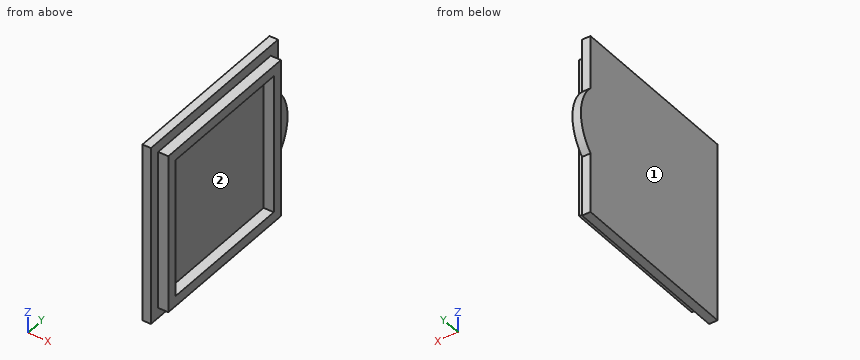
Autodesk Inventor part; units mm, degrees
ref_plane "YZ Plane" through (0, 0, 0) normal (1, 0, 0) x (0, 1, 0)
ref_plane "XZ Plane" through (0, 0, 0) normal (0, 1, 0) x (-1, 0, 0)
ref_plane "XY Plane" through (0, 0, 0) normal (0, 0, 1) x (1, 0, 0)
sketch "Skizze4" plane through (0, 0, 0) normal (1, 0, 0) x (0, 1, 0)
  line L0 (26.5, 26.5) -> (-26.5, 26.5)
  line L1 (-26.5, 26.5) -> (-26.5, -26.5)
  line L2 (-26.5, -26.5) -> (26.5, -26.5)
  line L3 (26.5, -26.5) -> (26.5, 26.5)
  line L4 (0, -37.1) -> (0, 37.1) construction
  line L5 (-37.1, 0) -> (37.1, 0) construction
  dimension "d18" = 53
  dimension "d19" = 53
extrude "Extrusion2" add sketch "Skizze4" along normal blind 2.5
sketch "Skizze5" plane through (2.5, 0, 0) normal (1, 0, 0) x (0, 0, -1)
  line L0 (-26.5, -26.5) -> (26.5, -26.5) construction
  line L1 (26.5, -26.5) -> (26.5, 26.5) construction
  line L2 (26.5, 26.5) -> (-26.5, 26.5) construction
  line L3 (-26.5, 26.5) -> (-26.5, -26.5) construction
  line L4 (-23.5, 23.5) -> (23.5, 23.5)
  line L5 (23.5, 23.5) -> (23.5, -23.5)
  line L6 (23.5, -23.5) -> (-23.5, -23.5)
  line L7 (-23.5, -23.5) -> (-23.5, 23.5)
  line L8 (20.5, 20.5) -> (-20.5, 20.5)
  line L9 (-20.5, 20.5) -> (-20.5, -20.5)
  line L10 (-20.5, -20.5) -> (20.5, -20.5)
  line L11 (20.5, -20.5) -> (20.5, 20.5)
  point P0 (0, 0)
  dimension "d8" = 3
  dimension "d9" = 3
extrude "Extrusion3" add sketch "Skizze5" along normal blind 3
sketch "Skizze6" plane through (0, 0, 0) normal (-1, 0, 0) x (0, 0, 1)
  line L0 (26.5, 26.5) -> (-26.5, 26.5) construction
  line L1 (26.5, -26.5) -> (26.5, 26.5) construction
  line L2 (-26.5, 26.5) -> (-26.5, 0) construction
  line L3 (0, -5.395) -> (0, 39.3226) construction
  line L4 (-26.5, 26.5) -> (26.5, 26.5)
  arc A0 (10.7474, 26.5) -> (-8.8486, 26.5) centre (0.9494, 16.5) ccw
  point P0 (0, 0)
  dimension "d12" = 26.5
  dimension "d13" = 53
  dimension "d14" = 14
  dimension "d15" = 10
extrude "Extrusion4" add sketch "Skizze6" against normal up to surface (2.5 mm away)
equation "\"d19\" = d18"
equation "\"d12\" = 0.5 * d13"
properties part number "Modul Deckel" material "Kst - PC/Makrolon (clear)"
Work out the finished part from the listing and answer in its coordinate system (mm). Face numbers are marked on the shaded views. Give positions to 0.01 mm unless a question says otherwise; leave off trailing zeros. Write each loop counter-clockwise with the first axis right and the second up, starting at its lowest first coordinate (ties: lowest second). Pieces come first, ordered by that corner, then holes.
(1) The mould has two halves that part along Z. Classify the marked faces 1 and 2: pulls with the +Z half, pulls with the -Z half, needs draft (parallel to the pull), parting line crosses it, or undercut.
Final values:
face 1: needs draft
face 2: undercut
(2) The part is cut by section C-C on x = 1.1. Write down the section's boundary in (y, z).
Final values:
outline: (-26.5, -26.5) - (26.5, -26.5) - (26.5, -8.85) arc R14 ccw to (26.5, 10.75) - (26.5, 26.5) - (-26.5, 26.5) - close
(3) The part is cut by section A-A on z = -22. Write down the section's boundary in (x, y).
Final values:
outline: (0, -26.5) - (2.5, -26.5) - (2.5, -23.5) - (5.5, -23.5) - (5.5, 23.5) - (2.5, 23.5) - (2.5, 26.5) - (0, 26.5) - close
(4) Straight lines are drawn through the part: line 1 (Z direction, x = 4.9, y = 16); line 2 (Y direction, x = 2.45, z = -19). For each, find the intervals that lie inside material, in ascending order.
Final values:
line 1: z = -23.5 to -20.5, 20.5 to 23.5
line 2: y = -26.5 to 26.5
(5) Flat-ended cylindrical pins translate along their axes: pin 1 Ø12 at (y, z) = (5, 5.5) entering from +X; pin 2 Ø0.9 at (x, z) = (4.5, -6.5) entering from -Y; pin 3 Ø1.2 at (x, z) = (1, -17.5) entering from +Y; pin 4 Ø12 at (y, z) = (-9, -3.5) entering from -X. Find the tip coordinate at first contact, or state that the pin passes through.
Final values:
pin 1: stops at x = 2.5
pin 2: stops at y = -23.5
pin 3: stops at y = 26.5
pin 4: stops at x = 0
(6) The part is cut by section D-D on y = 19. Write down the section's boundary in (x, z), plus the area to 4 significant figures.
Final values:
outline: (0, -26.5) - (2.5, -26.5) - (2.5, -23.5) - (5.5, -23.5) - (5.5, -20.5) - (2.5, -20.5) - (2.5, 20.5) - (5.5, 20.5) - (5.5, 23.5) - (2.5, 23.5) - (2.5, 26.5) - (0, 26.5) - close
area: 150.5 mm2
